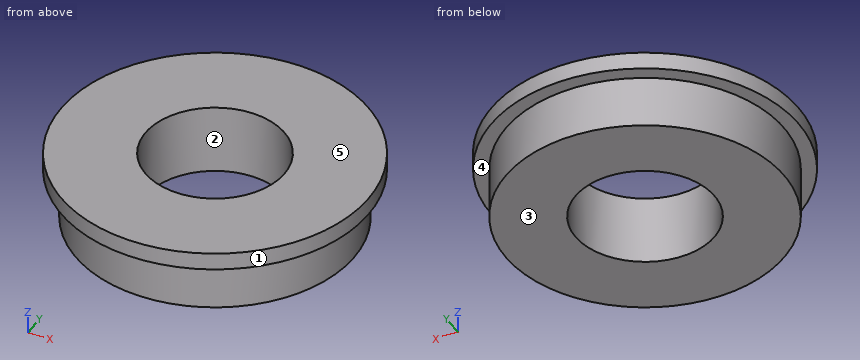
from build123d import *

# Parameters (mm, degrees)
SKETCH_1_R          = 12
EXTRUDE_1_DEPTH     = 4.5
SKETCH_2_R          = 13.25
EXTRUDE_2_DEPTH     = 1.5
SKETCH_3_R          = 6
CUT_EXTRUDE_1_DEPTH = 39.132990966


with BuildPart() as part:
    # ｽｹｯﾁ1 → 押し出し1 (new body)
    with BuildSketch(Plane.XY):
        with Locations((-22, 0)):
            Circle(SKETCH_1_R)
    extrude(amount=-EXTRUDE_1_DEPTH)

    # ｽｹｯﾁ2 → 押し出し2 (add)
    with BuildSketch(Plane.XY):
        with Locations((-22, 0)):
            Circle(SKETCH_2_R)
    extrude(amount=EXTRUDE_2_DEPTH)

    # ｽｹｯﾁ3 → ｶｯﾄ - 押し出し1 (cut, through all)
    with BuildSketch(Plane.XY.offset(1.5)):
        with Locations((-22, 0)):
            Circle(SKETCH_3_R)
    extrude(amount=-CUT_EXTRUDE_1_DEPTH, mode=Mode.SUBTRACT)


solid = part.part
The model under review builds one solid part; all positions refer to its coordinate system, in mm. Face numbers are marked on the shaded views. A direction names the side the tool comes from. Round coordinates to 2 decimals unless told otherwise and drop trailing zeros. Write each loop counter-clockwise with the first axis right and the second up, starting at its lowest first coordinate (ties: lowest second). Pieces come first, ordered by that corner, then holes. Notation, with made-up numbers: M -16,-35.5 L 11,-35.5 A17 ccw 11,-30.5 Z; hole C 41,20 d6. An arc over 180 degrees is marked long. Use a Markdown table: item, result. Add a question column.
Q1. Machinability: for the marked faces 4 and 5, which of the approach directions +Z, -Z, +X, -X, +Y, -Y give a long, thin tool a straight path to every point of the face, cutting with its end or side? Answer none if there is none.
Q2. To check wall thickness, follow line 1 (Y direction, x = -22, z = -1.8); line 2 (Y direction, x = -22, z = 0.1); line 3 (X direction, y = 4.75, z = 0.4). State the ranges of each line that lie inside material, in increasing order.
Q3. We need section A-A, the plane x = -22. State the section outline as (y, z) points, plus the area to 4 significant figures.
Q4. Insertion check: pin 1 (2 mm diameter, centred on x = -28, z = -2, fed in from -Y); pin 2 (1.5 mm diameter, centred on x = -12, z = -2.5, fed in from -Y); pin 3 (1.5 mm diameter, centred on y = -2.5, z = 0, fed in from +X). Each pin has a flat end and moves straight along its axis. Give the tip position at first contact, or say it passes through.
Q5. We need section D-D, the plane y = -7.75. State the section outline as (x, z) points.
Q6. The part is to be moulded in two halves that separate along Y. For the marked faces 1, 2 and 3, say which applies: pulls with the +Y half, pulls with the -Y half, needs draft (parallel to the pull), parting line crosses it, or undercut.
Q7. We need section B-B, the plane y = 0. State the section outline as (x, z) points, plus the area to 4 significant figures.
Q8. We need section C-C, the plane z = -3. State the section outline as (x, y) points, plus the area to 3 significant figures.
Findings below:
| question | item | result |
|---|---|---|
| 1 | face 4 | -Z |
| 1 | face 5 | +Z, +X, -X, +Y, -Y |
| 2 | line 1 | y = -12 to -6, 6 to 12 |
| 2 | line 2 | y = -13.25 to -6, 6 to 13.25 |
| 2 | line 3 | x = -34.37 to -25.67, -18.33 to -9.63 |
| 3 | outline | M -13.25,0 L -12,0 L -12,-4.5 L -6,-4.5 L -6,1.5 L -13.25,1.5 Z; M 6,-4.5 L 12,-4.5 L 12,0 L 13.25,0 L 13.25,1.5 L 6,1.5 Z |
| 3 | area | 75.75 mm² |
| 4 | pin 1 | stops at y = -10.91 |
| 4 | pin 2 | stops at y = -7.64 |
| 4 | pin 3 | stops at x = -8.87 |
| 5 | outline | M -32.75,0 L -31.16,0 L -31.16,-4.5 L -12.84,-4.5 L -12.84,0 L -11.25,0 L -11.25,1.5 L -32.75,1.5 Z |
| 6 | face 1 | parting line crosses it |
| 6 | face 2 | undercut |
| 6 | face 3 | needs draft |
| 7 | outline | M -35.25,0 L -34,0 L -34,-4.5 L -28,-4.5 L -28,1.5 L -35.25,1.5 Z; M -16,-4.5 L -10,-4.5 L -10,0 L -8.75,0 L -8.75,1.5 L -16,1.5 Z |
| 7 | area | 75.75 mm² |
| 8 | outline | C -22,0 d24; hole C -22,0 d12 |
| 8 | area | 339 mm² |
